```python
from build123d import *

# Parameters (mm, degrees)
BOSS_EXTRUDE1_DEPTH = 31.75
BOSS_EXTRUDE2_REACH = 148.188
CUT_EXTRUDE1_DEPTH  = 53.975


with BuildPart() as part:
    # Sketch1 → Boss-Extrude1 (new, symmetric)
    with BuildSketch(Plane(origin=(0, 0, 0), x_dir=(0, 0, -1), z_dir=(1, 0, 0))):
        with BuildLine():
            Line((0, 0), (-133.35, 0))
            Line((-133.35, 0), (-133.35, 16.898297196))
            ThreePointArc((-133.35, 16.898297196), (-132.748070755, 18.540089432), (-131.227573428, 19.403737762))
            Line((-131.227573428, 19.403737762), (-77.389477645, 28.376753726))
            ThreePointArc((-77.389477645, 28.376753726), (-76.355301792, 28.797962054), (-75.601713492, 29.622001389))
            Line((-75.601713492, 29.622001389), (-64.231318341, 49.520192903))
            ThreePointArc((-64.231318341, 49.520192903), (-63.300874878, 50.456871637), (-62.02598076, 50.8))
            Line((-62.02598076, 50.8), (-45.916469684, 50.8))
            ThreePointArc((-45.916469684, 50.8), (-44.646469684, 50.459704526), (-43.716765158, 49.53))
            Line((-43.716765158, 49.53), (-23.186189586, 13.97))
            ThreePointArc((-23.186189586, 13.97), (-22.25648506, 13.040295474), (-20.98648506, 12.7))
            Line((-20.98648506, 12.7), (-2.54, 12.7))
            ThreePointArc((-2.54, 12.7), (-0.743948776, 11.956051224), (0, 10.16))
            Line((0, 10.16), (0, 0))
        make_face()
    extrude(amount=BOSS_EXTRUDE1_DEPTH, both=True)

    # Sketch2 → Boss-Extrude2 (add, up to next)
    with BuildSketch(Plane(origin=(0, 0, 0), x_dir=(-1, 0, 0), z_dir=(0, 0, -1)), mode=Mode.PRIVATE) as boss_extrude2_sk1:
        with BuildLine():
            Line((-31.75, 0), (-12.7, 0))
            Line((-12.7, 0), (12.7, 0))
            Line((12.7, 0), (31.75, 0))
            Line((31.75, 0), (31.75, 10.16))
            Line((31.75, 10.16), (25.4, 10.16))
            ThreePointArc((25.4, 10.16), (0, 35.56), (-25.4, 10.16))
            Line((-25.4, 10.16), (-31.75, 10.16))
            Line((-31.75, 10.16), (-31.75, 0))
        make_face()
    boss_extrude2_tool1 = extrude(boss_extrude2_sk1.sketch, amount=-BOSS_EXTRUDE2_REACH, mode=Mode.PRIVATE) - part.part
    add(boss_extrude2_tool1.solids().sort_by_distance((0, 14.770763, 0))[0])

    # Sketch3 → Cut-Extrude1 (cut)
    with BuildSketch(Plane(origin=(0, 0, 0), x_dir=(-1, 0, 0), z_dir=(0, 0, -1))):
        with BuildLine():
            Line((-12.7, 0), (12.7, 0))
            Line((12.7, 0), (12.7, 12.7))
            ThreePointArc((12.7, 12.7), (0, 25.4), (-12.7, 12.7))
            Line((-12.7, 12.7), (-12.7, 0))
        make_face()
    extrude(amount=-CUT_EXTRUDE1_DEPTH, mode=Mode.SUBTRACT)


solid = part.part
```
Read the model definition and answer for the solid it produces. Units are mm, in the model's axes. A direction names the side the tool comes from. Give positions to 0.01 mm unless a question says otherwise; leave off trailing zeros. Write each loop counter-clockwise with the first axis right and the second up, starting at its lowest first coordinate (ties: lowest second). Pieces come first, ordered by that corner, then holes. Notation, with made-up numbers: (22, 69.5) -> (63, 69.5) arc R10 cw to (63, 80.5) -> close; hole circle Ø11 at (15.5, 7.25). An arc over 180 degrees is marked (long way). Answer as a JSON object with one key per item and string values.
1) Section A-A on x = 0 is taken. Write down the section's boundary in (y, z) (3 decimals), then the cut area to 3 significant figures.
Findings below:
{"outline": "(0, 53.975) -> (25.4, 53.975) -> (25.4, 0) -> (35.56, 0) -> (35.56, 35.651) -> (49.53, 43.717) arc R2.54 ccw to (50.8, 45.916) -> (50.8, 62.026) arc R2.54 ccw to (49.52, 64.231) -> (29.622, 75.602) arc R2.54 cw to (28.377, 77.389) -> (19.404, 131.228) arc R2.54 ccw to (16.898, 133.35) -> (0, 133.35) -> close", "area": "3,110 mm^2"}
2) Section B-B on y = 33.5 is taken. Write down the section's boundary in (x, z), then the cut area to 3 significant figures.
Findings below:
{"outline": "(-31.75, 34.46) -> (-10.02, 34.46) -> (-10.02, 0) -> (10.02, 0) -> (10.02, 34.46) -> (31.75, 34.46) -> (31.75, 73.39) -> (-31.75, 73.39) -> close", "area": "3,160 mm^2"}
3) Straight lines are drawn through the part: probe 1 along X at (y, z) = (12.5, 17.5); probe 2 along Z at (x, y) = (-11.5, 3.5) (3 decimals); probe 3 along Y at (x, z) = (-21.5, 78.5). For each, find the intervals that lie inside material, in ascending order. Write a range as from..to.
Findings below:
{"probe 1": "x = -31.75..-12.7, 12.7..31.75", "probe 2": "z = 53.975..133.35", "probe 3": "y = 0..28.19"}
4) Section D-D on x = -27 is taken. Write down the section's boundary in (y, z).
Findings below:
{"outline": "(0, 0) -> (10.16, 0) arc R2.54 ccw to (12.7, 2.54) -> (12.7, 20.99) arc R2.54 cw to (13.97, 23.19) -> (49.53, 43.72) arc R2.54 ccw to (50.8, 45.92) -> (50.8, 62.03) arc R2.54 ccw to (49.52, 64.23) -> (29.62, 75.6) arc R2.54 cw to (28.38, 77.39) -> (19.4, 131.23) arc R2.54 ccw to (16.9, 133.35) -> (0, 133.35) -> close"}
5) Section C-C on z = 29 is taken. Write down the section's boundary in (x, y), then the cut area to 3 significant figures.
Findings below:
{"outline": "(-31.75, 0) -> (-12.7, 0) -> (-12.7, 12.7) arc R12.7 cw to (12.7, 12.7) -> (12.7, 0) -> (31.75, 0) -> (31.75, 24.04) -> (21.27, 24.04) arc R25.4 ccw to (-21.27, 24.04) -> (-31.75, 24.04) -> close", "area": "1,300 mm^2"}
6) A tool of negligible diameter and unlimited length cuts with its end or side. For faces 1 (the cylindrical face through (-0.559, 35.554, 13.615)), 2 (the flat face through (31.75, 14, 66)), 3 (the cylindrical face through (-0.279, 25.397, 26.61)), 4 (the flat face through (-28, 12.7, 12)), 5 (the cylindrical face through (28.557, 11.976, 0.764)), from which of +Z, -Z, +X, -X, +Y, -Y can it reach the whole face along a straight path? Write none if from no direction.
Findings below:
{"face 1": "-Z, +Y", "face 2": "+Z, -Z, +X, +Y, -Y", "face 3": "-Z, -Y", "face 4": "-Z, -X, +Y", "face 5": "-Z, +X, +Y"}
7) Flat-ended cylindrical pins translate along their axes: pin 1 Ø5 at (x, z) = (29.5, 16) entering from +Y; pin 2 Ø12.5 at (x, y) = (1, 19) entering from -Z (3 decimals); pin 3 Ø5 at (x, z) = (-6.5, 98) entering from +Y; pin 4 Ø6 at (x, y) = (17, 25) entering from -Z. Find the tip coordinate at first contact, or state that the pin passes through.
Findings below:
{"pin 1": "stops at y = 12.7", "pin 2": "stops at z = 53.975", "pin 3": "stops at y = 25.36", "pin 4": "stops at z = 0"}
